For this review, use the dimensioned drawing (mm, ordinates from the lowest corner) and the shaded views. A direction names the side the tool comes from. Coordinates: 2 decimals unless noted, no trailing zeros. Write each loop counter-clockwise with the first axis right and the second up, starting at its lowest first coordinate (ties: lowest second). Pieces come first, ordered by that corner, then holes.
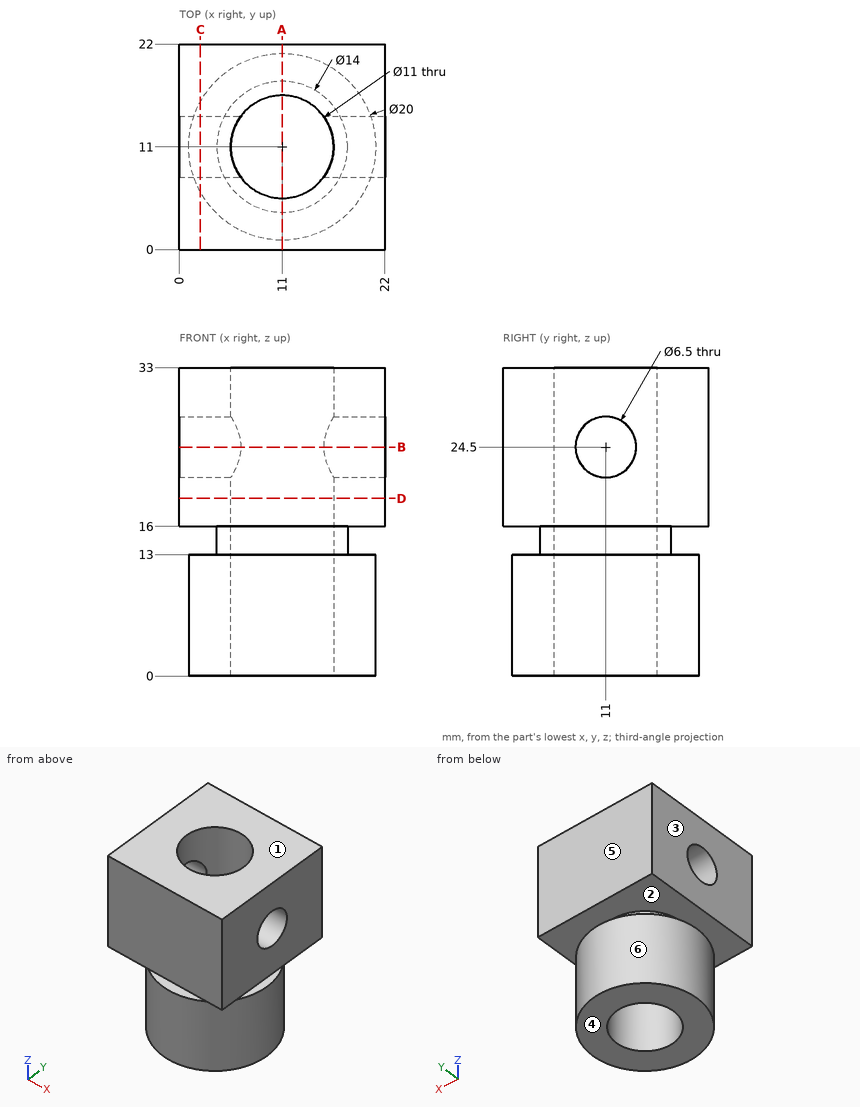
(1) Consider section D-D (z = 19). Give the boundary of the cut face in (x, y).
(2) Insertion check: pin 1 Ø6 at (y, z) = (11, 24.5) entering from -X. The pin has a flat end and moves straight along its axis. Give the tip position at first contact, or say it passes through.
(3) Mouldability with a two-part tool opening along Z and no side actions: class the marked faces 1, 2, 3 and 4 as +Z half, -Z half, draft (parallel to the pull), parting line (faces both ways), or undercut.
(4) For the marked faces 5 and 6, list the 3-axis set-ups (+Z, -Z, +X, -X, +Y, -Y) from which the entire face can be reached by the end or side of a thin tool; tool diameter is ignored.
(5) Wall thickness on line 1 (Z direction, x = 18.75, y = 11); line 2 (Y direction, x = 11, z = 20); line 3 (Y direction, x = 10.75, z = 10): over which ranges is each line inside the solid? List them lowest first.
(6) Consider section C-C (x = 2.25). Give the boundary of the cut face in (y, z), plus the area to 3 significant figures.
(7) Consider section A-A (x = 11). Give the boundary of the cut face in (y, z).
(8) Consider section B-B (z = 24.5). Give the boundary of the cut face in (x, y), plus the area to 3 significant figures.
Results:
1. outline: (0, 0) - (22, 0) - (22, 22) - (0, 22) - close; hole circle Ø11 at (11, 11)
2. pin 1: passes through
3. face 1: +Z half
3. face 2: undercut
3. face 3: draft
3. face 4: -Z half
4. face 5: +Z, -Z, +X, -X, +Y
4. face 6: -Z
5. line 1: z = 0 to 13, 16 to 21.25, 27.75 to 33
5. line 2: y = 0 to 5.5, 16.5 to 22
5. line 3: y = 1 to 5.51, 16.49 to 21
6. outline: (0, 16) - (22, 16) - (22, 33) - (0, 33) - close; (6.16, 0) - (15.84, 0) - (15.84, 13) - (6.16, 13) - close; hole circle Ø6.5 at (11, 24.5)
6. area: 467 mm2
7. outline: (0, 16) - (4, 16) - (4, 13) - (1, 13) - (1, 0) - (5.5, 0) - (5.5, 33) - (0, 33) - close; (16.5, 0) - (21, 0) - (21, 13) - (18, 13) - (18, 16) - (22, 16) - (22, 33) - (16.5, 33) - close
8. outline: (0, 0) - (22, 0) - (22, 7.75) - (15.44, 7.75) arc R5.5 cw to (6.56, 7.75) - (0, 7.75) - close; (0, 14.25) - (6.56, 14.25) arc R5.5 cw to (15.44, 14.25) - (22, 14.25) - (22, 22) - (0, 22) - close
8. area: 313 mm2
